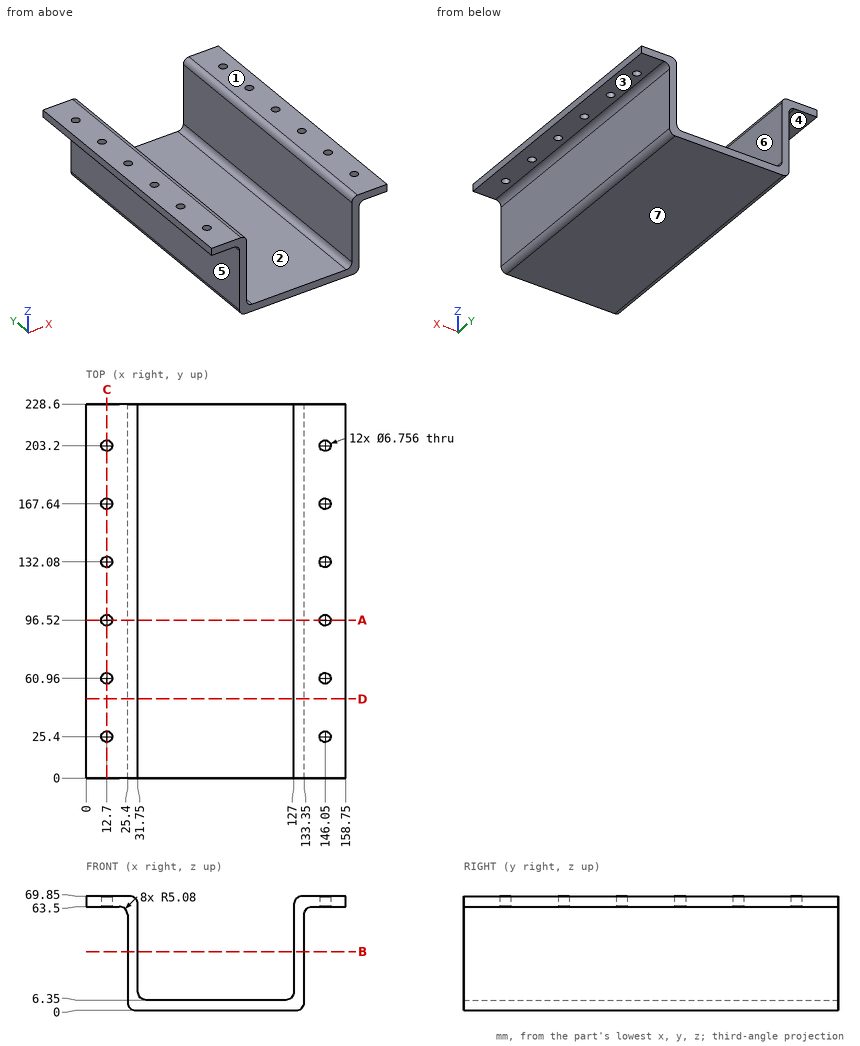
Could you check a few things on this drawing? It's one solid part, dimensions in mm from its lowest x, y, z. A direction names the side the tool comes from. Coordinates: 2 decimals unless noted, no trailing zeros. Loops run counter-clockwise (first coordinate to the right, second up) from the corner with the lowest first, then second, coordinate; pieces in that order, holes last.
1. Imagine slicing it at D-D (y = 48.5). Please give me the cut outline in (x, z), and give its area (3 significant figures).
2. Imagine slicing it at C-C (x = 12.7). Please give me the cut outline in (y, z).
3. Imagine slicing it at B-B (z = 36). Please give me the cut outline in (x, y).
4. Imagine slicing it at A-A (y = 96.52). Please give me the cut outline in (x, z), and give its area (3 significant figures).
5. For P1, Ø1, axis at y = 101, z = 49, coming from the +X side; P2, Ø22.5, axis at x = 7, y = 139, coming from the -Z side; P3, Ø2, axis at x = 115.5, y = 115, coming from the -Z side; P4, Ø4, axis at y = 115, z = 34.5, coming from the -X side, each with a flat end and sliding along its axis, tell me the tip position at first contact or that it passes through.
6. We'd pull the mould along X, two halves only. Please class the marked faces 5, 6 and 7: released by +X, released by -X, zero draft, split by the parting line, or undercut.
7. For the marked faces 1, 2, 3 and 4, which set-ups out of +Z, -Z, +X, -X, +Y, -Y let a thin tool reach every point of the face, with its end or its side?
8. I need wall thicknesses on L1, parallel to X at y = 97, z = 51; L2, parallel to Z at x = 18, y = 43.5; L3, parallel to Z at x = 43, y = 143.5. Which ranges of each line are inside material? Lowest first, please.
Computed values:
1. outline: (0, 63.5) - (20.32, 63.5) arc R5.08 cw to (25.4, 58.42) - (25.4, 5.08) arc R5.08 ccw to (30.48, 0) - (128.27, 0) arc R5.08 ccw to (133.35, 5.08) - (133.35, 58.42) arc R5.08 cw to (138.43, 63.5) - (158.75, 63.5) - (158.75, 69.85) - (132.08, 69.85) arc R5.08 ccw to (127, 64.77) - (127, 11.43) arc R5.08 cw to (121.92, 6.35) - (36.83, 6.35) arc R5.08 cw to (31.75, 11.43) - (31.75, 64.77) arc R5.08 ccw to (26.67, 69.85) - (0, 69.85) - close
1. area: 1,810 mm2
2. outline: (0, 63.5) - (22.02, 63.5) - (22.02, 69.85) - (0, 69.85) - close; (28.78, 63.5) - (57.58, 63.5) - (57.58, 69.85) - (28.78, 69.85) - close; (64.34, 63.5) - (93.14, 63.5) - (93.14, 69.85) - (64.34, 69.85) - close; (99.9, 63.5) - (128.7, 63.5) - (128.7, 69.85) - (99.9, 69.85) - close; (135.46, 63.5) - (164.26, 63.5) - (164.26, 69.85) - (135.46, 69.85) - close; (171.02, 63.5) - (199.82, 63.5) - (199.82, 69.85) - (171.02, 69.85) - close; (206.58, 63.5) - (228.6, 63.5) - (228.6, 69.85) - (206.58, 69.85) - close
3. outline: (25.4, 0) - (31.75, 0) - (31.75, 228.6) - (25.4, 228.6) - close; (127, 0) - (133.35, 0) - (133.35, 228.6) - (127, 228.6) - close
4. outline: (0, 63.5) - (9.32, 63.5) - (9.32, 69.85) - (0, 69.85) - close; (16.08, 63.5) - (20.32, 63.5) arc R5.08 cw to (25.4, 58.42) - (25.4, 5.08) arc R5.08 ccw to (30.48, 0) - (128.27, 0) arc R5.08 ccw to (133.35, 5.08) - (133.35, 58.42) arc R5.08 cw to (138.43, 63.5) - (142.67, 63.5) - (142.67, 69.85) - (132.08, 69.85) arc R5.08 ccw to (127, 64.77) - (127, 11.43) arc R5.08 cw to (121.92, 6.35) - (36.83, 6.35) arc R5.08 cw to (31.75, 11.43) - (31.75, 64.77) arc R5.08 ccw to (26.67, 69.85) - (16.08, 69.85) - close; (149.43, 63.5) - (158.75, 63.5) - (158.75, 69.85) - (149.43, 69.85) - close
4. area: 1,730 mm2
5. P1: stops at x = 133.35
5. P2: stops at z = 63.5
5. P3: stops at z = 0
5. P4: stops at x = 25.4
6. face 5: released by -X
6. face 6: undercut
6. face 7: zero draft
7. face 1: +Z, +X, -X, +Y, -Y
7. face 2: +Z, +Y, -Y
7. face 3: -Z, +X, +Y, -Y
7. face 4: -Z, -X, +Y, -Y
8. L1: x = 25.4 to 31.75, 127 to 133.35
8. L2: z = 63.5 to 69.85
8. L3: z = 0 to 6.35
